Check sheet for the modelled part. Datum: model origin and axes. Units: mm. Face numbers are marked on the shaded views. A direction names the side the tool comes from. Coordinates: 2 decimals unless noted, no trailing zeros. Loops run counter-clockwise (first coordinate to the right, second up) from the corner with the lowest first, then second, coordinate; pieces in that order, holes last. Notation, with made-up numbers: (70.25, -25) -> (95.25, -25) arc R24 ccw to (95.25, 8) -> close; hole circle Ø6 at (-17, 24.5). An arc over 180 degrees is marked (long way). Use CSV: the item, a comma, the result in double quotes.
```python
from build123d import *

# Parameters (mm, degrees)
SKETCH1_R           = 17.5
SKETCH1_R_2         = 15.5
BOSS_EXTRUDE1_DEPTH = 5
SKETCH3_R           = 17.5
BOSS_EXTRUDE2_DEPTH = 4
SKETCH2_R           = 16.9
SKETCH2_R_2         = 16.1
CUT_EXTRUDE1_DEPTH  = 8


with BuildPart() as part:
    # Sketch1 → Boss-Extrude1 (new body)
    with BuildSketch(Plane(origin=(0, 0, 0), x_dir=(1, 0, 0), z_dir=(0, 1, 0))):
        Circle(SKETCH1_R)
        Circle(SKETCH1_R_2, mode=Mode.SUBTRACT)
    extrude(amount=BOSS_EXTRUDE1_DEPTH)

    # Sketch3 → Boss-Extrude2 (add)
    with BuildSketch(Plane.XZ):
        Circle(SKETCH3_R)
        with BuildLine():
            ThreePointArc((-0.299732076, 3.537323944), (-2.510229073, 2.510229073), (-3.537323944, 0.299732076))
            ThreePointArc((-3.537323944, 0.299732076), (-3.25, 0), (-3.537323944, -0.299732076))
            ThreePointArc((-3.537323944, -0.299732076), (-2.510229073, -2.510229073), (-0.299732076, -3.537323944))
            ThreePointArc((-0.299732076, -3.537323944), (0, -3.25), (0.299732076, -3.537323944))
            ThreePointArc((0.299732076, -3.537323944), (2.510229073, -2.510229073), (3.537323944, -0.299732076))
            ThreePointArc((3.537323944, -0.299732076), (3.25, 0), (3.537323944, 0.299732076))
            ThreePointArc((3.537323944, 0.299732076), (2.510229073, 2.510229073), (0.299732076, 3.537323944))
            ThreePointArc((0.299732076, 3.537323944), (0, 3.25), (-0.299732076, 3.537323944))
        make_face(mode=Mode.SUBTRACT)
    extrude(amount=BOSS_EXTRUDE2_DEPTH)

    # Sketch2 → Cut-Extrude1 (cut)
    with BuildSketch(Plane(origin=(0, 5, 0), x_dir=(1, 0, 0), z_dir=(0, 1, 0))):
        Circle(SKETCH2_R)
        Circle(SKETCH2_R_2, mode=Mode.SUBTRACT)
    extrude(amount=-CUT_EXTRUDE1_DEPTH, mode=Mode.SUBTRACT)


solid = part.part
```
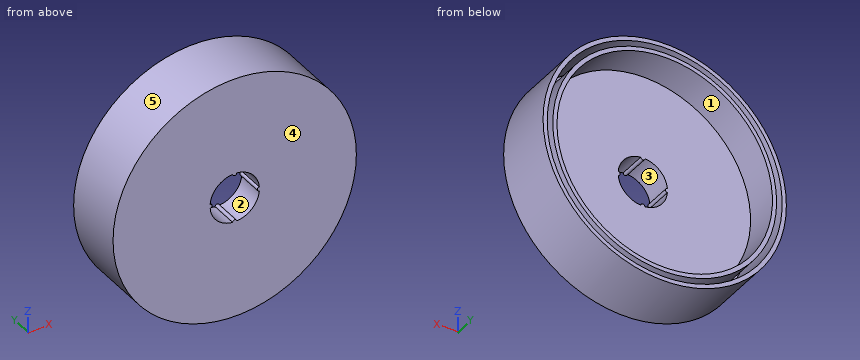
1) Access from +Z, -Z, +X, -X, +Y, -Y to the whole of each face (thin tool, end or side, straight path). Record for the marked faces 1 and 2.
Answer below:
face 1,"+Y"
face 2,"+Y, -Y"
2) Thickness scan on line 1 along X through (y, z) = (2.5, 0); line 2 along X through (y, z) = (-2.5, -14); line 3 along Z through (x, y) = (-3.5, 0.25). Record the ranges inside material, lowest first. Write a range as from..to.
Answer below:
line 1,"x = -17.5..-16.9, -16.1..-15.5, 15.5..16.1, 16.9..17.5"
line 2,"x = -10.5..-9.47, -7.95..7.95, 9.47..10.5"
line 3,"z = -17.15..-16.53, -15.71..-15.1, 15.1..15.71, 16.53..17.15"
3) Go/stop test with flat-tipped pins: pin 1 Ø1.5 at (x, y) = (-13, 3) entering from -Z; pin 2 Ø9.5 at (x, z) = (7.5, -5.5) entering from +Y; pin 3 Ø1 at (y, z) = (0.5, -6.5) entering from +X. Record where each tip stops, or that it passes through.
Answer below:
pin 1,"stops at z = -12.5"
pin 2,"stops at y = 0"
pin 3,"stops at x = 16.44"
4) Cross-section at C-C on x = -11. Record the boundary of the cut face in (y, z), and give its area (3 significant figures).
Answer below:
outline,"(-4, -13.61) -> (5, -13.61) -> (5, -12.83) -> (-3, -12.83) -> (-3, -11.76) -> (5, -11.76) -> (5, -10.92) -> (0, -10.92) -> (0, 10.92) -> (5, 10.92) -> (5, 11.76) -> (-3, 11.76) -> (-3, 12.83) -> (5, 12.83) -> (5, 13.61) -> (-4, 13.61) -> close"
area,"119 mm²"
5) Cross-section at B-B on z = -1. Record the boundary of the cut face in (x, y), and give its area (3 significant figures).
Answer below:
outline,"(-17.47, -4) -> (-3.41, -4) -> (-3.41, 0) -> (-15.47, 0) -> (-15.47, 5) -> (-16.07, 5) -> (-16.07, -3) -> (-16.87, -3) -> (-16.87, 5) -> (-17.47, 5) -> close; (3.41, -4) -> (17.47, -4) -> (17.47, 5) -> (16.87, 5) -> (16.87, -3) -> (16.07, -3) -> (16.07, 5) -> (15.47, 5) -> (15.47, 0) -> (3.41, 0) -> close"
area,"120 mm²"
6) Cross-section at D-D on y = 2.5. Record the boundary of the cut face in (x, z), and give its area (3 significant figures).
Answer below:
outline,"circle Ø35 at (0, 0); circle Ø32.2 at (0, 0); hole circle Ø33.8 at (0, 0); hole circle Ø31 at (0, 0)"
area,"124 mm²"
7) Cross-section at A-A on y = -0.75. Record the boundary of the cut face in (x, z), and give its area (3 significant figures).
Answer below:
outline,"circle Ø35 at (0, 0); circle Ø32.2 at (0, 0); hole circle Ø33.8 at (0, 0); hole (-3.54, -0.3) arc R3.55 ccw to (-0.3, -3.54) arc R0.3 cw to (0.3, -3.54) arc R3.55 ccw to (3.54, -0.3) arc R0.3 cw to (3.54, 0.3) arc R3.55 ccw to (0.3, 3.54) arc R0.3 cw to (-0.3, 3.54) arc R3.55 ccw to (-3.54, 0.3) arc R0.3 cw to start"
area,"840 mm²"
8) Draft check along X on the marked faces 3, 4 and 5. Enter one of: released by +X, released by -X, zero draft, split by the parting line, or undercut.
Answer below:
face 3,"undercut"
face 4,"zero draft"
face 5,"split by the parting line"
